Build history of the part. All positions in model axes, mm. Face numbers are marked on the shaded views. A direction names the side the tool comes from. Round coordinates to 2 decimals unless told otherwise and drop trailing zeros. Write each loop counter-clockwise with the first axis right and the second up, starting at its lowest first coordinate (ties: lowest second). Pieces come first, ordered by that corner, then holes.
1) Which spindle directions (+Z, -Z, +X, -X, +Y, -Y) get a long thin tool onto all of the face, cutting with end or side? Do the marked faces 1 and 2. Say none if no direction does.
2) Pull direction X, two halves, no side cores. Call the marked faces 3, 4 and 5: +X half, -X half, draft (parallel to the pull), parting line (faces both ways), or undercut.
3) Wall check: probe 1 along Z at (x, y) = (1, -11.25); probe 2 along X at (y, z) = (-15.5, 0.5); probe 3 along Z at (x, y) = (0, -3.9). Give the ranges that are in metal, low to high.
4) Saw through at C-C (y = -11). Write the cut outline in (x, z).
5) Saw through at B-B (x = 0). Write the cut outline in (y, z), plus the area to 3 significant figures.
6) Saw through at A-A (z = 0). Write the cut outline in (x, y).
7) Flat gauge pins, fed straight in: pin 1 (1 mm diameter, centred on x = -23, y = -8, fed in from +Z); pin 2 (10 mm diameter, centred on x = -9.5, y = -4, fed in from -Z); pin 3 (10 mm diameter, centred on x = 9, z = 9, fed in from +Y); pin 4 (2 mm diameter, centred on y = -10.5, z = 24, fed in from +X). Where does each tip first touch, or does it go through?
from build123d import *

# Parameters (mm, degrees)
F0_R     = 34.5
F1_DEPTH = 18.5
F2_R     = 27.5
F3_DEPTH = 10
F4_R     = 29.5
F5_DEPTH = 6
F6_R     = 19.5
F7_DEPTH = 2.501
F8_SIZE  = 1


with BuildPart() as f1:
    # F0 (on Front) → F1 (new body)
    with BuildSketch(Plane.XZ):
        Circle(F0_R)
    extrude(amount=F1_DEPTH)

    # F2 (on face) → F3 (cut)
    with BuildSketch(Plane.XZ.offset(18.5)):
        Circle(F2_R)
    extrude(amount=-F3_DEPTH, mode=Mode.SUBTRACT)

    # F4 (on face) → F5 (cut)
    with BuildSketch(Plane.XZ.offset(8.5)):
        Circle(F4_R)
    extrude(amount=-F5_DEPTH, mode=Mode.SUBTRACT)

    # F6 (on face) → F7 (cut, through all)
    with BuildSketch(Plane.XZ.offset(2.5)):
        Circle(F6_R)
    extrude(amount=-F7_DEPTH, mode=Mode.SUBTRACT)

    # F8
    f8_edges = [f1.edges().sort_by_distance(p)[0] for p in [
        (-34.5, -18.5, 0),
        (-27.5, -18.5, 0),
        (-34.5, 0, 0),
    ]]
    chamfer(f8_edges, length=F8_SIZE)


solid = f1.part
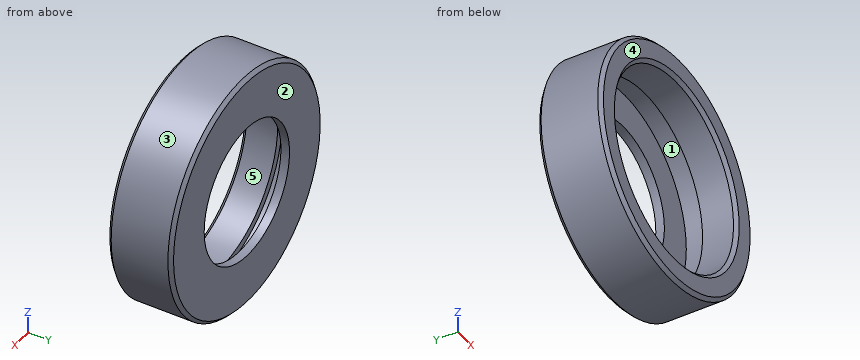
Evaluation:
1. face 1: none
1. face 2: +Z, -Z, +X, -X, +Y
2. face 3: parting line
2. face 4: draft
2. face 5: undercut
3. probe 1: z = -34.49 to -27.48, 27.48 to 34.49
3. probe 2: x = -34.5 to -27.5, 27.5 to 34.5
3. probe 3: z = -34.5 to -29.5, 29.5 to 34.5
4. outline: circle Ø69 at (0, 0); hole circle Ø55 at (0, 0)
5. outline: (-18.5, -33.5) - (-17.5, -34.5) - (-1, -34.5) - (0, -33.5) - (0, -19.5) - (-2.5, -19.5) - (-2.5, -29.5) - (-8.5, -29.5) - (-8.5, -27.5) - (-17.5, -27.5) - (-18.5, -28.5) - close; (-18.5, 28.5) - (-17.5, 27.5) - (-8.5, 27.5) - (-8.5, 29.5) - (-2.5, 29.5) - (-2.5, 19.5) - (0, 19.5) - (0, 33.5) - (-1, 34.5) - (-17.5, 34.5) - (-18.5, 33.5) - close
5. area: 272 mm2
6. outline: (-34.5, -17.5) - (-33.5, -18.5) - (-28.5, -18.5) - (-27.5, -17.5) - (-27.5, -8.5) - (-29.5, -8.5) - (-29.5, -2.5) - (-19.5, -2.5) - (-19.5, 0) - (-33.5, 0) - (-34.5, -1) - close; (19.5, -2.5) - (29.5, -2.5) - (29.5, -8.5) - (27.5, -8.5) - (27.5, -17.5) - (28.5, -18.5) - (33.5, -18.5) - (34.5, -17.5) - (34.5, -1) - (33.5, 0) - (19.5, 0) - close
7. pin 1: stops at z = 26.15
7. pin 2: stops at z = -34.21
7. pin 3: passes through
7. pin 4: stops at x = 25.71
